from build123d import *

# Parameters (mm, degrees)
BOSS_EXTRUDE1_DEPTH = 25
SKETCH2_W           = 5.5
SKETCH2_H           = 36
CUT_EXTRUDE1_DEPTH  = 31.396710348
SKETCH3_R           = 1.6
CUT_EXTRUDE2_DEPTH  = 31.396710348


with BuildPart() as part:
    # Sketch1 → Boss-Extrude1 (new, symmetric)
    with BuildSketch(Plane(origin=(0, 0, 0), x_dir=(1, 0, 0), z_dir=(0, 1, 0))):
        Polygon((7.5, 0), (-7.5, 0), (-7.5, -3), (-3.9, -3), (-3.9, -13), (-0.9, -13), (-0.9, -7), (0.9, -7), (0.9, -13), (3.9, -13), (3.9, -3), (7.5, -3), align=None)
    extrude(amount=BOSS_EXTRUDE1_DEPTH, both=True)

    # Sketch2 → Cut-Extrude1 (cut, through all)
    with BuildSketch(Plane.ZY.offset(3.9)):
        with Locations((10.25, 0)):
            Rectangle(SKETCH2_W, SKETCH2_H)
    extrude(amount=-CUT_EXTRUDE1_DEPTH, mode=Mode.SUBTRACT)

    # Sketch3 → Cut-Extrude2 (cut, through all)
    with BuildSketch(Plane.ZY.offset(3.9)):
        with Locations((9.5, 22.5)):
            Circle(SKETCH3_R)
        with Locations((9.5, -21)):
            Circle(SKETCH3_R)
    extrude(amount=-CUT_EXTRUDE2_DEPTH, mode=Mode.SUBTRACT)


solid = part.part
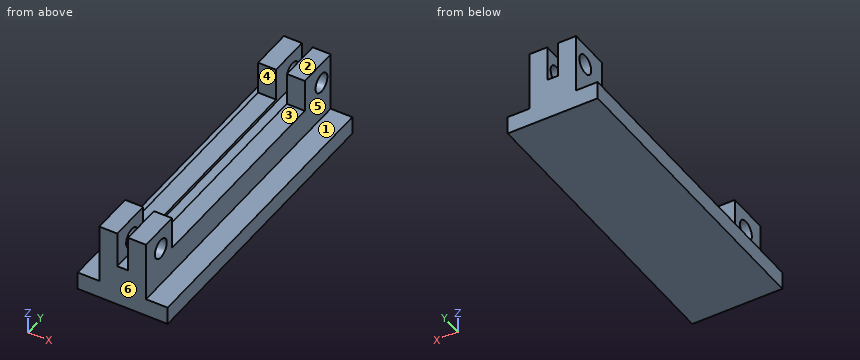
Could you check a few things on this model? Use its own coordinates, in mm. Face numbers are marked on the shaded views. A direction names the side the tool comes from. Round coordinates to 2 decimals unless told otherwise and drop trailing zeros. Loops run counter-clockwise (first coordinate to the right, second up) from the corner with the lowest first, then second, coordinate; pieces in that order, holes last. Notation, with made-up numbers: (-2, 57.5) -> (5, 57.5) arc R5 ccw to (5, 62.5) -> close; hole circle Ø4 at (-19, -21). An arc over 180 degrees is marked (long way). Use CSV: the item, a comma, the result in double quotes.
(1) For the marked faces 1, 2 and 3, which set-ups out of +Z, -Z, +X, -X, +Y, -Y let a thin tool reach every point of the face, with its end or its side?
Return value:
face 1,"+Z, +X, +Y, -Y"
face 2,"+Z, +X, -X, +Y, -Y"
face 3,"+Z, +X, -X"
(2) Will these pins go through, and if not, where does the flat tip stop? pin 1 Ø1 at (x, z) = (-5, 8.5) entering from -Y; pin 2 Ø0.9 at (x, y) = (3, 1) entering from +Z; pin 3 Ø6.5 at (y, z) = (11, 10) entering from -X; pin 4 Ø1.8 at (x, y) = (5.5, -12.5) entering from +Z.
Return value:
pin 1,"passes through"
pin 2,"stops at z = 7.5"
pin 3,"stops at x = -3.9"
pin 4,"stops at z = 3"
(3) If we mould it in two halves opening along Y, with no side actions, what happens to the marked faces 4, 5 and 6? For each: +Y half, -Y half, draft (parallel to the pull), parting line (faces both ways), or undercut.
Return value:
face 4,"undercut"
face 5,"draft"
face 6,"-Y half"
(4) Suppose I cut it at D-D on y = -21. Write out the boundary of the cut face in (x, z).
Return value:
outline,"(-7.5, 0) -> (7.5, 0) -> (7.5, 3) -> (3.9, 3) -> (3.9, 7.9) -> (0.9, 7.9) -> (0.9, 7) -> (-0.9, 7) -> (-0.9, 7.9) -> (-3.9, 7.9) -> (-3.9, 3) -> (-7.5, 3) -> close; (-3.9, 11.1) -> (-0.9, 11.1) -> (-0.9, 13) -> (-3.9, 13) -> close; (0.9, 11.1) -> (3.9, 11.1) -> (3.9, 13) -> (0.9, 13) -> close"
(5) Suppose I cut it at C-C on x = -1.75. Write out the boundary of the cut face in (y, z), plus the area to 3 significant figures.
Return value:
outline,"(-25, 0) -> (25, 0) -> (25, 13) -> (18, 13) -> (18, 7.5) -> (-18, 7.5) -> (-18, 13) -> (-25, 13) -> close; hole circle Ø3.2 at (-21, 9.5); hole circle Ø3.2 at (22.5, 9.5)"
area,"436 mm²"
(6) If I drill on probe 1 along Y at (x, z) = (-3.1, 9.5); probe 2 along Z at (x, y) = (5.25, -1); probe 3 along X at (y, z) = (-13.5, 5.25), over which ranges is the centre line in solid material (lowest first)? Write a range as [from, to].
Return value:
probe 1,"y = [-25, -22.6], [-19.4, -18], [18, 20.9], [24.1, 25]"
probe 2,"z = [0, 3]"
probe 3,"x = [-3.9, 3.9]"
(7) Suppose I cut it at A-A on z = 9.5. Give the number of separate pieces and of enclosed holes in the cut face, plus the area to 3 significant figures.
Return value:
separate pieces,"8"
enclosed holes,"0"
area,"45.6 mm²"
(8) Suppose I cut it at B-B on z = 12.25. Write out the boundary of the cut face in (x, y), plus the area to 3 significant figures.
Return value:
outline,"(-3.9, -25) -> (-0.9, -25) -> (-0.9, -18) -> (-3.9, -18) -> close; (-3.9, 18) -> (-0.9, 18) -> (-0.9, 25) -> (-3.9, 25) -> close; (0.9, -25) -> (3.9, -25) -> (3.9, -18) -> (0.9, -18) -> close; (0.9, 18) -> (3.9, 18) -> (3.9, 25) -> (0.9, 25) -> close"
area,"84.0 mm²"
